```python
from build123d import *

# Parameters (mm, degrees)
F1_DEPTH = 4.7625
F3_D     = 11.1125
F4_D     = 7.9375


# Not quite as in the source:
# - a length typed as a fraction of an inch, garbled in the dataset ("3 / 203.2 mm" for 3/8 in), is restored


with BuildPart() as f1:
    # F0 (on Top) → F1 (new body, symmetric)
    with BuildSketch(Plane.XY):
        with BuildLine():
            ThreePointArc((533.4, 88.9), (469.9, 128.5875), (406.4, 88.9))
            Line((406.4, 88.9), (-406.4, 88.9))
            ThreePointArc((-406.4, 88.9), (-469.9, 128.5875), (-533.4, 88.9))
            Line((-533.4, 88.9), (-533.4, -88.9))
            ThreePointArc((-533.4, -88.9), (-469.9, -128.5875), (-406.4, -88.9))
            Line((-406.4, -88.9), (406.4, -88.9))
            ThreePointArc((406.4, -88.9), (469.9, -128.5875), (533.4, -88.9))
            Line((533.4, -88.9), (533.4, 88.9))
        make_face()
        Polygon((-364.33125, -64.29375), (-228.6, -7.9375), (-92.86875, -64.29375), align=None, mode=Mode.SUBTRACT)
        Polygon((189.70625, -64.29375), (279.4, -7.9375), (369.09375, -64.29375), align=None, mode=Mode.SUBTRACT)
        with BuildLine():
            ThreePointArc((-487.3625, 88.9), (-484.98125, 91.28125), (-482.6, 88.9))
            Line((-482.6, 88.9), (-482.6, -88.9))
            ThreePointArc((-482.6, -88.9), (-484.98125, -91.28125), (-487.3625, -88.9))
            Line((-487.3625, -88.9), (-487.3625, 88.9))
        make_face(mode=Mode.SUBTRACT)
        with BuildLine():
            ThreePointArc((-457.2, 88.9), (-454.81875, 91.28125), (-452.4375, 88.9))
            Line((-452.4375, 88.9), (-452.4375, -88.9))
            ThreePointArc((-452.4375, -88.9), (-454.81875, -91.28125), (-457.2, -88.9))
            Line((-457.2, -88.9), (-457.2, 88.9))
        make_face(mode=Mode.SUBTRACT)
        Polygon((-381, -56.35625), (-381, 56.35625), (-245.26875, 0), align=None, mode=Mode.SUBTRACT)
        Polygon((-76.2, -56.35625), (-211.93125, 0), (-76.2, 56.35625), align=None, mode=Mode.SUBTRACT)
        Polygon((-92.86875, 63.5), (-228.6, 7.14375), (-364.33125, 63.5), align=None, mode=Mode.SUBTRACT)
        Polygon((177.8, 56.35625), (267.49375, 0), (177.8, -56.35625), align=None, mode=Mode.SUBTRACT)
        Polygon((291.30625, 0), (381, 56.35625), (381, -56.35625), align=None, mode=Mode.SUBTRACT)
        with BuildLine():
            Line((452.4375, -88.9), (452.4375, 88.9))
            ThreePointArc((452.4375, 88.9), (454.81875, 91.28125), (457.2, 88.9))
            Line((457.2, 88.9), (457.2, -88.9))
            ThreePointArc((457.2, -88.9), (454.81875, -91.28125), (452.4375, -88.9))
        make_face(mode=Mode.SUBTRACT)
        with BuildLine():
            ThreePointArc((487.3625, -88.9), (484.98125, -91.28125), (482.6, -88.9))
            Line((482.6, -88.9), (482.6, 88.9))
            ThreePointArc((482.6, 88.9), (484.98125, 91.28125), (487.3625, 88.9))
            Line((487.3625, 88.9), (487.3625, -88.9))
        make_face(mode=Mode.SUBTRACT)
        Polygon((369.09375, 63.5), (279.4, 7.14375), (189.70625, 63.5), align=None, mode=Mode.SUBTRACT)
    extrude(amount=F1_DEPTH, both=True)

    # F3 (through all)
    with Locations(Plane.XY.offset(4.7625)):
        with Locations((0, 50.8), (101.6, 50.8), (101.6, -50.8), (0, -50.8)):
            Hole(F3_D / 2)

    # F4 (through all)
    with Locations(Plane.XY.offset(4.7625)):
        with Locations((-46.83125, 30.1625), (-46.83125, -30.1625), (11.1125, 16.69415), (91.28125, 16.69415), (148.43125, 30.1625), (148.43125, -30.1625)):
            Hole(F4_D / 2)


solid = f1.part
```
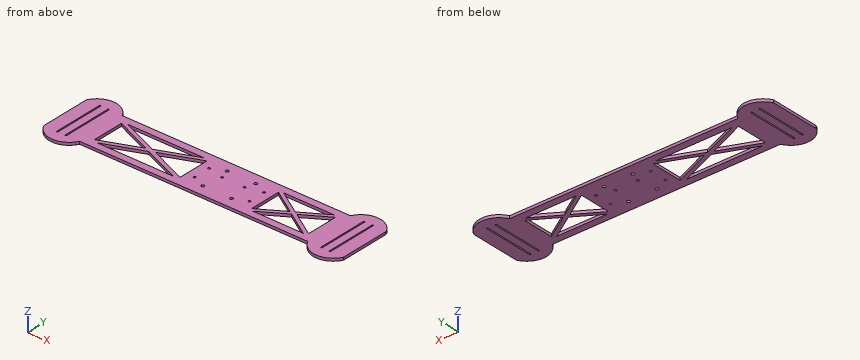
Model file for the job. Use its own axes, mm. Give positions to 0.01 mm unless a question says otherwise; leave off trailing zeros. Write each loop counter-clockwise with the first axis right and the second up, starting at its lowest first coordinate (ties: lowest second). Pieces come first, ordered by that corner, then holes. Notation, with made-up numbers: (-39.75, -6) -> (-30.75, -6) arc R8 ccw to (-30.75, 9) -> close; hole circle Ø8 at (25, 1.5). An arc over 180 degrees is marked (long way). Use CSV: the item, a comma, the result in double quotes. Start each with the question number.
1) Drill centre lines: L1, parallel to Y at x = 0, z = -1.5; L2, parallel to X at y = -70.5, z = -2; L3, parallel to Y at x = 237.5, z = 2. Where is each one in solid material? Low to high.
2) Cut at C-C on z = -1.5. Count the separate pieces of the cut face and the enclosed holes in it, plus the area to 3 significant figures.
3) Cut at D-D on x = 77.5. List the corners of the cut face in (y, z), plus the area to 3 significant figures.
4) Cut at A-A on y = 79. List the corners of the cut face in (x, z), plus the area to 3 significant figures.
5) Cut at B-B on x = 207. List the corners of the cut face in (y, z).
6) Pin check, flat tip, straight feed: P1, Ø1, axis at y = 102, z = 1.5, coming from the +X side. Stop position of the tip, or through.
Final values:
1,L1,"y = -88.9 to -56.36, -45.24 to 45.24, 56.36 to 88.9"
1,L2,"x = -533.4 to -487.36, -482.6 to -457.2, -452.44 to 452.44, 457.2 to 482.6, 487.36 to 533.4"
1,L3,"y = -88.9 to -64.29, -34.26 to -18.85, 18.85 to 33.47, 63.5 to 88.9"
2,separate pieces,"1"
2,enclosed holes,"22"
2,area,"149,000 mm2"
3,outline,"(-88.9, -4.76) -> (88.9, -4.76) -> (88.9, 4.76) -> (-88.9, 4.76) -> close"
3,area,"1,690 mm2"
4,outline,"(-533.4, -4.76) -> (-487.36, -4.76) -> (-487.36, 4.76) -> (-533.4, 4.76) -> close; (-482.6, -4.76) -> (-457.2, -4.76) -> (-457.2, 4.76) -> (-482.6, 4.76) -> close; (-452.44, -4.76) -> (452.44, -4.76) -> (452.44, 4.76) -> (-452.44, 4.76) -> close; (457.2, -4.76) -> (482.6, -4.76) -> (482.6, 4.76) -> (457.2, 4.76) -> close; (487.36, -4.76) -> (533.4, -4.76) -> (533.4, 4.76) -> (487.36, 4.76) -> close"
4,area,"9,980 mm2"
5,outline,"(-88.9, -4.76) -> (-64.29, -4.76) -> (-64.29, 4.76) -> (-88.9, 4.76) -> close; (-53.43, -4.76) -> (-38.01, -4.76) -> (-38.01, 4.76) -> (-53.43, 4.76) -> close; (38.01, -4.76) -> (52.63, -4.76) -> (52.63, 4.76) -> (38.01, 4.76) -> close; (63.5, -4.76) -> (88.9, -4.76) -> (88.9, 4.76) -> (63.5, 4.76) -> close"
6,P1,"stops at x = 525.52"
